Geometry: final body of the model. Coordinates: model frame, mm. Face numbers are marked on the shaded views. A direction names the side the tool comes from. Give positions to 0.01 mm unless a question says otherwise; leave off trailing zeros. Write each loop counter-clockwise with the first axis right and the second up, starting at its lowest first coordinate (ties: lowest second). Pieces come first, ordered by that corner, then holes. Notation, with made-up numbers: (-23.5, -5.75) -> (9.5, -5.75) arc R17 cw to (9.5, 6.25) -> close; hole circle Ø11 at (53.5, 70.25). An arc over 180 degrees is marked (long way). Answer in a Markdown table with one row per item. Add a question column.
Item 1: Material intervals for probe 1 along X at (y, z) = (5.75, -19.05) (3 decimals); probe 2 along Z at (x, y) = (16.5, 23.5) (3 decimals); probe 3 along Z at (x, y) = (33, 3), sorted ascending. Write a range as from..to.
Item 2: Section query D-D on y = 3. Output: boundary loops of the cut face in (x, z) (3 decimals), plus the area to 3 significant figures.
Item 3: Section query B-B on y = 31. Output: boundary loops of the cut face in (x, z) (3 decimals).
Item 4: Draft query along Z for the marked faces 3, 4, 5 and 6. Return one class per face: +Z half, -Z half, draft (parallel to the pull), parting line (faces both ways), or undercut.
Item 5: Section query C-C on x = 5. Output: boundary loops of the cut face in (y, z) (3 decimals).
Item 6: Access query for the marked faces 1 and 2. Directions: +Z, -Z, +X, -X, +Y, -Y. A direction counts if a zero-diameter tool reaches every point of the face in a straight line with its end or side. Return the directions, or none.
Item 7: Section query A-A on z = -19.05. Output: boundary loops of the cut face in (x, y) (3 decimals), plus the area to 3 significant figures.
Item 8: First-contact query: P1, Ø5.5, axis at x = 10.922, z = -19.05, coming from the -Y side; P2, Ø2, axis at x = 30, z = -29.5, coming from the +Y side (3 decimals). Flat tips, straight axial feed; report the tip coordinate or a pass-through.
```python
from build123d import *

# Parameters (mm, degrees)
SKETCH1_W           = 42.672
SKETCH1_H           = 38.1
BOSS_EXTRUDE1_DEPTH = 7.62
SKETCH3_R           = 3.175
CUT_EXTRUDE1_DEPTH  = 7.62
SKETCH4_R           = 10.922
SKETCH4_R_2         = 3.175
BOSS_EXTRUDE2_DEPTH = 9.525
FILLET1_START       = -9.525
FILLET1_DEPTH       = 9.525
FILLET2_R           = 6.35
FILLET3_R           = 6.35


with BuildPart() as part:
    # Sketch1 → Boss-Extrude1 (new body)
    with BuildSketch(Plane(origin=(0, 0, 0), x_dir=(1, 0, 0), z_dir=(0, 1, 0))):
        with Locations((21.336, 19.05)):
            Rectangle(SKETCH1_W, SKETCH1_H)
    extrude(amount=BOSS_EXTRUDE1_DEPTH)

    # Sketch3 → Cut-Extrude1 (cut)
    with BuildSketch(Plane(origin=(0, 7.62, 0), x_dir=(-1, 0, 0), z_dir=(0, 1, 0))):
        with Locations(Location((-10.922, -19.05, 0), (0, 0, 90))):
            Circle(SKETCH3_R)
        with Locations(Location((-33.02, -19.05, 0), (0, 0, 90))):
            Circle(SKETCH3_R)
    extrude(amount=-CUT_EXTRUDE1_DEPTH, mode=Mode.SUBTRACT)

    # Sketch4 → Boss-Extrude2 (add)
    # profile 1 of 2: a face of its own
    with BuildSketch(Plane.XY):
        with BuildLine():
            Line((0, 27.178), (0, 7.62))
            Line((0, 7.62), (21.844, 7.62))
            Line((21.844, 7.62), (21.844, 27.178))
            ThreePointArc((21.844, 27.178), (10.922, 16.256), (0, 27.178))
        make_face()
    # profile 2 of 2: a face of its own
    with BuildSketch(Plane.XY):
        with Locations((10.922, 27.178)):
            Circle(SKETCH4_R)
        with Locations((10.922, 27.178)):
            Circle(SKETCH4_R_2, mode=Mode.SUBTRACT)
    boss_extrude2 = extrude(amount=-BOSS_EXTRUDE2_DEPTH)

    # Fillet1: read off the stored shape, not the designer's step
    # Fillet1 outline → Fillet1 (add)
    with BuildSketch(Plane.XY.offset(FILLET1_START)):
        with BuildLine():
            Line((21.844, 7.62), (41.402, 7.62))
            add(Edge.make_bspline(
                [(41.402, 7.62), (21.844, 7.62), (21.844, 27.178)],
                knots=[0, 0, 0, 1, 1, 1], degree=2, weights=[1, 0.707106781, 1]))
            Line((21.844, 27.178), (21.844, 7.62))
        make_face()
    fillet1 = extrude(amount=FILLET1_DEPTH)

    # Fillet2
    fillet2_edges = [part.edges().sort_by_distance(p)[0] for p in [
        (42.672, 3.81, 0),
    ]]
    fillet(fillet2_edges, radius=FILLET2_R)

    # Mirror2: Boss-Extrude2, Fillet1 across plane
    add(boss_extrude2.mirror(Plane.XY.offset(-19.05)))
    add(fillet1.mirror(Plane.XY.offset(-19.05)))

    # Fillet3
    fillet3_edges = [part.edges().sort_by_distance(p)[0] for p in [
        (42.672, 3.81, -38.1),
    ]]
    fillet(fillet3_edges, radius=FILLET3_R)


solid = part.part
```
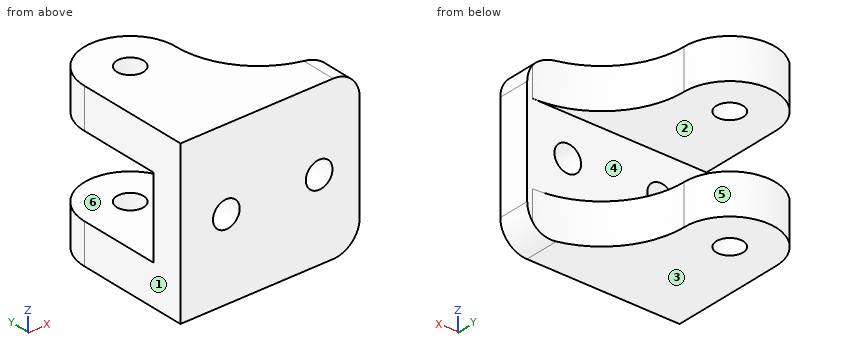
Findings below:
| question | item | result |
|---|---|---|
| 1 | probe 1 | x = 0..7.747, 14.097..29.845, 36.195..42.672 |
| 1 | probe 2 | z = -38.1..-28.575, -9.525..0 |
| 1 | probe 3 | z = -38.1..-22.22, -15.88..0 |
| 2 | outline | (0, -38.1) -> (36.322, -38.1) arc R6.35 ccw to (42.672, -31.75) -> (42.672, -6.35) arc R6.35 ccw to (36.322, 0) -> (0, 0) -> close; hole circle Ø6.35 at (10.922, -19.05); hole circle Ø6.35 at (33.02, -19.05) |
| 2 | area | 1,550 mm^2 |
| 3 | outline | (0.691, -38.1) -> (21.153, -38.1) -> (21.153, -28.575) -> (0.691, -28.575) -> close; (0.691, -9.525) -> (21.153, -9.525) -> (21.153, 0) -> (0.691, 0) -> close |
| 4 | face 3 | -Z half |
| 4 | face 4 | undercut |
| 4 | face 5 | draft |
| 4 | face 6 | undercut |
| 5 | outline | (0, -38.1) -> (36.355, -38.1) -> (36.355, -28.575) -> (7.62, -28.575) -> (7.62, -9.525) -> (36.355, -9.525) -> (36.355, 0) -> (0, 0) -> close |
| 6 | face 1 | +Z, -Z, -X, +Y, -Y |
| 6 | face 2 | +X, -X, +Y |
| 7 | outline | (0, 0) -> (7.747, 0) -> (7.747, 7.62) -> (0, 7.62) -> close; (14.097, 0) -> (29.845, 0) -> (29.845, 7.62) -> (14.097, 7.62) -> close; (36.195, 0) -> (42.672, 0) -> (42.672, 7.62) -> (36.195, 7.62) -> close |
| 7 | area | 228 mm^2 |
| 8 | P1 | passes through |
| 8 | P2 | stops at y = 12.055 |
